Autodesk Inventor part; units mm, degrees
ref_plane "작업 평면1" through (0, 2.2, 0) normal (0, 1, 0) x (1, 0, 0)
ref_plane "YZ Plane" through (0, 0, 0) normal (1, 0, 0) x (0, 1, 0)
ref_plane "XZ Plane" through (0, 0, 0) normal (0, 1, 0) x (-1, 0, 0)
sketch "스케치1" plane through (0, 0, 0) normal (0, 1, 0) x (-1, 0, 0)
  line L0 (12.4723, -12.4723) -> (4.5652, -17.0375)
  line L1 (4.5652, -17.0375) -> (-4.5652, -17.0375)
  line L2 (-4.5652, -17.0375) -> (-12.4723, -12.4723)
  line L3 (-12.4723, -12.4723) -> (-17.0375, -4.5652)
  line L4 (-17.0375, -4.5652) -> (-17.0375, 4.5652)
  line L5 (-17.0375, 4.5652) -> (-12.4723, 12.4723)
  line L6 (-12.4723, 12.4723) -> (-4.5652, 17.0375)
  line L7 (-4.5652, 17.0375) -> (4.5652, 17.0375)
  line L8 (4.5652, 17.0375) -> (12.4723, 12.4723)
  line L9 (12.4723, 12.4723) -> (17.0375, 4.5652)
  line L10 (17.0375, 4.5652) -> (17.0375, -4.5652)
  line L11 (17.0375, -4.5652) -> (12.4723, -12.4723)
  line L12 (-5.4226, 20.2375) -> (5.4226, 20.2375)
  line L13 (5.4226, 20.2375) -> (14.8149, 14.8149)
  line L14 (14.8149, 14.8149) -> (20.2375, 5.4226)
  line L15 (20.2375, 5.4226) -> (20.2375, -5.4226)
  line L16 (20.2375, -5.4226) -> (14.8149, -14.8149)
  line L17 (14.8149, -14.8149) -> (5.4226, -20.2375)
  line L18 (5.4226, -20.2375) -> (-5.4226, -20.2375)
  line L19 (-5.4226, -20.2375) -> (-14.8149, -14.8149)
  line L20 (-14.8149, -14.8149) -> (-20.2375, -5.4226)
  line L21 (-20.2375, -5.4226) -> (-20.2375, 5.4226)
  line L22 (-20.2375, 5.4226) -> (-14.8149, 14.8149)
  line L23 (-14.8149, 14.8149) -> (-5.4226, 20.2375)
  point P0 (0, 0)
  point P1 (0, 0)
  point P2 (0, 0)
  dimension "d0" = 35.277
  dimension "d1" = 3.2
extrude "돌출1" add sketch "스케치1" along normal blind 4.4 contours L0 L1 L2 L3 L4 L5 L6 L7 L8 L9 L10 L11 | L12 L13 L14 L15 L16 L17 L18 L19 L20 L21 L22 L23
fillet "모깎기1" radius 1.2 24 edges at (10.1187, 4.4, 17.5262) (17.5262, 4.4, 10.1187) (20.2375, 4.4, 0) (17.5262, 4.4, -10.1187) (10.1187, 4.4, -17.5262) (0, 4.4, -20.2375) (-10.1187, 4.4, -17.5262) (-17.5262, 4.4, -10.1187) (-20.2375, 4.4, 0) (-17.5262, 4.4, 10.1187) (-10.1187, 4.4, 17.5262) (0, 4.4, 20.2375) (-10.1187, 0, 17.5262) (-17.5262, 0, 10.1187) (-20.2375, 0, 0) (-10.1187, 0, -17.5262) (-17.5262, 0, -10.1187) (0, 0, -20.2375) (10.1187, 0, -17.5262) (17.5262, 0, -10.1187) (20.2375, 0, 0) (17.5262, 0, 10.1187) (10.1187, 0, 17.5262) (0, 0, 20.2375)
sketch "스케치6" plane through (0, 0, 0) normal (0, -1, 0) x (1, 0, 0)
  line L0 (13.6436, -13.6436) -> (4.9939, -18.6375)
  line L1 (4.9939, -18.6375) -> (-4.9939, -18.6375)
  line L2 (-4.9939, -18.6375) -> (-13.6436, -13.6436)
  line L3 (-13.6436, -13.6436) -> (-18.6375, -4.9939)
  line L4 (-18.6375, -4.9939) -> (-18.6375, 4.9939)
  line L5 (-18.6375, 4.9939) -> (-13.6436, 13.6436)
  line L6 (-13.6436, 13.6436) -> (-4.9939, 18.6375)
  line L7 (-4.9939, 18.6375) -> (4.9939, 18.6375)
  line L8 (4.9939, 18.6375) -> (13.6436, 13.6436)
  line L9 (13.6436, 13.6436) -> (18.6375, 4.9939)
  line L10 (18.6375, 4.9939) -> (18.6375, -4.9939)
  line L11 (18.6375, -4.9939) -> (13.6436, -13.6436)
  line L12 (20.2375, 5.4226) -> (14.8149, 14.8149)
  line L13 (4.458, 16.6375) -> (12.1795, 12.1795)
  line L14 (12.1795, 12.1795) -> (16.6375, 4.458)
  line L15 (16.6375, 4.458) -> (16.6375, -4.458)
  line L16 (16.6375, -4.458) -> (12.1795, -12.1795)
  line L17 (12.1795, -12.1795) -> (4.458, -16.6375)
  line L18 (4.458, -16.6375) -> (-4.458, -16.6375)
  line L19 (-4.458, -16.6375) -> (-12.1795, -12.1795)
  line L20 (-12.1795, -12.1795) -> (-16.6375, -4.458)
  line L21 (-16.6375, -4.458) -> (-16.6375, 4.458)
  line L22 (-16.6375, 4.458) -> (-12.1795, 12.1795)
  line L23 (-12.1795, 12.1795) -> (-4.458, 16.6375)
  line L24 (-4.458, 16.6375) -> (4.458, 16.6375)
  point P0 (0, 0)
  point P1 (0, 0)
  point P2 (0, 0)
  dimension "d20" = 1.6
  dimension "d21" = 2
extrude "돌출6" cut sketch "스케치6" against normal blind 1.2
sketch "스케치7" plane through (0, 0, 0) normal (0, -1, 0) x (1, 0, 0)
  line L0 (16.6375, 4.458) -> (12.1795, 12.1795)
  line L1 (12.1795, 12.1795) -> (4.458, 16.6375)
  line L2 (4.458, 16.6375) -> (-4.458, 16.6375)
  line L3 (-4.458, 16.6375) -> (-12.1795, 12.1795)
  line L4 (-12.1795, 12.1795) -> (-16.6375, 4.458)
  line L5 (-16.6375, 4.458) -> (-16.6375, -4.458)
  line L6 (-16.6375, -4.458) -> (-12.1795, -12.1795)
  line L7 (-12.1795, -12.1795) -> (-4.458, -16.6375)
  line L8 (-4.458, -16.6375) -> (4.458, -16.6375)
  line L9 (4.458, -16.6375) -> (12.1795, -12.1795)
  line L10 (12.1795, -12.1795) -> (16.6375, -4.458)
  line L11 (16.6375, -4.458) -> (16.6375, 4.458)
  point P0 (0, 0)
extrude "돌출7" cut sketch "스케치7" against normal blind 0.6
ref_plane "작업 평면1" through (0, 2.2, 0) normal (0, 1, 0) x (1, 0, 0)
mirror "미러1" about plane through (0, 2.2, 0) normal (0, 1, 0) of "돌출7", "돌출6"
sketch "스케치10" plane through (-4.458, 3.8, -16.6375) normal (0, 1, 0) x (1, 0, 0)
  line L0 (0.3215, -32.075) -> (-6.843, -27.9385)
  line L1 (-6.843, -27.9385) -> (-10.9795, -20.7739)
  line L2 (-10.9795, -20.7739) -> (-10.9795, -12.501)
  line L3 (-10.9795, -12.501) -> (-6.843, -5.3365)
  line L4 (-6.843, -5.3365) -> (0.3215, -1.2)
  line L5 (0.3215, -1.2) -> (8.5945, -1.2)
  line L6 (8.5945, -1.2) -> (15.759, -5.3365)
  line L7 (15.759, -5.3365) -> (19.8955, -12.501)
  line L8 (19.8955, -12.501) -> (19.8955, -20.7739)
  line L9 (19.8955, -20.7739) -> (15.759, -27.9385)
  line L10 (15.759, -27.9385) -> (8.5945, -32.075)
  line L11 (8.5945, -32.075) -> (0.3215, -32.075)
  line L12 (8.916, -33.275) -> (0, -33.275)
  point P0 (4.458, -16.6375)
  point P1 (4.458, -16.6375)
  dimension "d37" = 1.2
extrude "돌출10" cut sketch "스케치10" against normal blind 10
properties part number "(x0.5)_POSPA_Tiny_Top"
Geometry: final body of the model. Coordinates: model frame, mm. A direction names the side the tool comes from. Give positions to 0.01 mm unless a question says otherwise; leave off trailing zeros. Write each loop counter-clockwise with the first axis right and the second up, starting at its lowest first coordinate (ties: lowest second). Pieces come first, ordered by that corner, then holes.
(1) First-contact query: P1, Ø16.5, axis at x = 0.5, z = -8, coming from the -Y side; P2, Ø1.3, axis at y = 4, z = -1.5, coming from the -X side. Flat tips, straight axial feed; report the tip coordinate or a pass-through.
(2) Mould query, pull axis X, two halves, no side actions, for faces 4 (the cylindrical face through (-17.3, 4, 9.9)), 5 (the flat face through (-14.44, 0.896, 8.265)), 6 (the cylindrical face through (0.076, 4.039, -19.895)), 7 (the flat face through (20.238, 2, 0)). Classes: released by +X, released by -X, zero draft, split by the parting line, or undercut.
(3) Ray query, line 1 (Z direction, x = 4, y = 3.35); line 2 (Z direction, x = -14, y = 0.8); line 3 (X direction, y = 0.7, z = -2). Return the intervals inside material, ascending.
(4) Access query for faces 1 (the flat face through (0, 1, -18.638)), 2 (the flat face through (-7.77, 2.22, -13.34)), 3 (the flat face through (9.258, 3.808, -16.176)). Directions: +Z, -Z, +X, -X, +Y, -Y. A direction counts if a zero-diameter tool reaches every point of the face in a straight line with its end or side. Return the directions, or none.
(5) Cut plane B-B, the plane y = 2.55. Return loops of the section in (x, z), then the cut area to 3 significant figures.
(6) Cut plane A-A, the plane x = 2. Return loops of the section in (y, z), then the cut area to 3 significant figures.
Values follow:
1. P1: stops at y = 0.6
1. P2: stops at x = -20.23
2. face 4: released by -X
2. face 5: undercut
2. face 6: zero draft
2. face 7: released by +X
3. line 1: z = -20.23 to -18.64, -16.64 to -15.44, 15.44 to 16.64, 18.64 to 20.23
3. line 2: z = -15.21 to -13.03, -9.03 to -6.63, 6.63 to 9.03, 13.03 to 15.21
3. line 3: x = -20.13 to -18.64, -16.64 to -15.44, 15.44 to 16.64, 18.64 to 20.13
4. face 1: -Y
4. face 2: +Y, -Y
4. face 3: +Y
5. outline: (-20.24, -5.42) - (-14.81, -14.81) - (-5.42, -20.24) - (5.42, -20.24) - (14.81, -14.81) - (20.24, -5.42) - (20.24, 5.42) - (14.81, 14.81) - (5.42, 20.24) - (-5.42, 20.24) - (-14.81, 14.81) - (-20.24, 5.42) - close; hole (-15.44, -4.14) - (-11.3, -11.3) - (-4.14, -15.44) - (4.14, -15.44) - (11.3, -11.3) - (15.44, -4.14) - (15.44, 4.14) - (11.3, 11.3) - (4.14, 15.44) - (-4.14, 15.44) - (-11.3, 11.3) - (-15.44, 4.14) - close
5. area: 551 mm2
6. outline: (0, -19.04) arc R1.2 ccw to (1.2, -20.24) - (3.2, -20.24) arc R1.2 ccw to (4.4, -19.04) - (4.4, -18.64) - (3.2, -18.64) - (3.2, -16.64) - (3.8, -16.64) - (3.8, -15.44) - (0.6, -15.44) - (0.6, -16.64) - (1.2, -16.64) - (1.2, -18.64) - (0, -18.64) - close; (0, 18.64) - (1.2, 18.64) - (1.2, 16.64) - (0.6, 16.64) - (0.6, 15.44) - (3.8, 15.44) - (3.8, 16.64) - (3.2, 16.64) - (3.2, 18.64) - (4.4, 18.64) - (4.4, 19.04) arc R1.2 ccw to (3.2, 20.24) - (1.2, 20.24) arc R1.2 ccw to (0, 19.04) - close
6. area: 28.5 mm2
